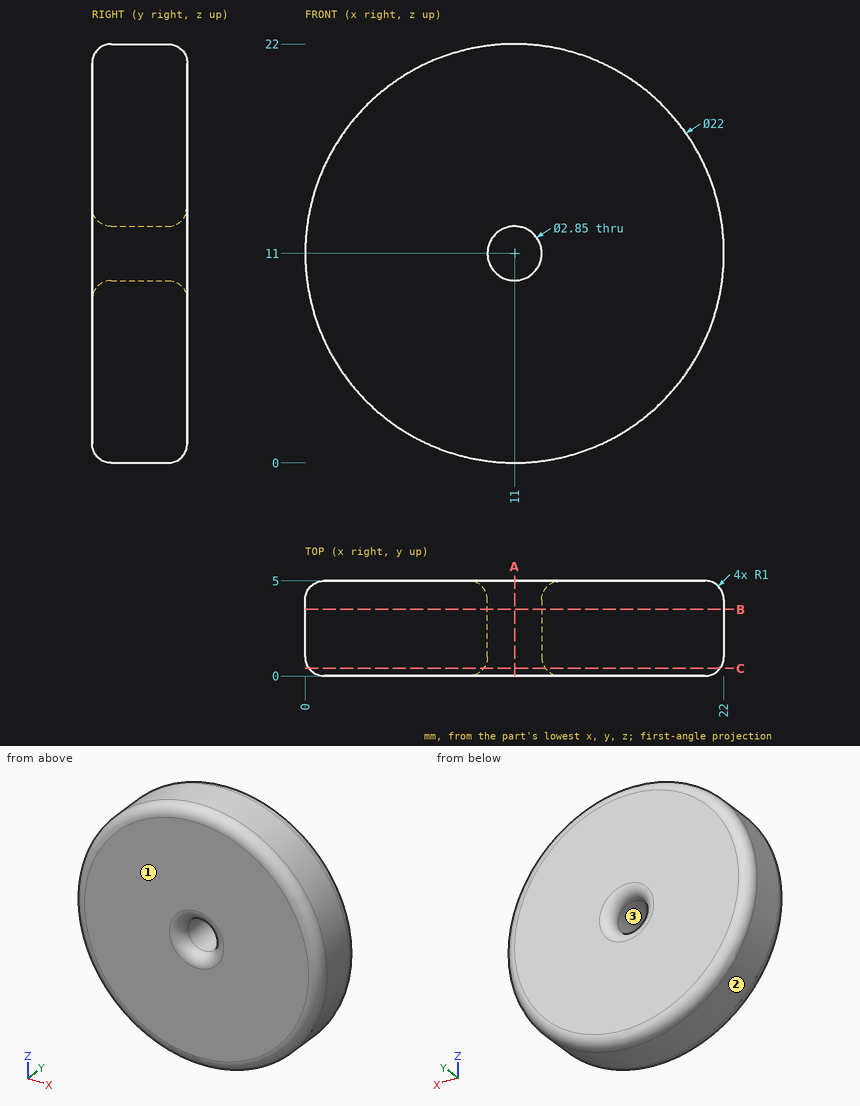
Here's the drawing with two shaded views (mm, measured from the low corner). I have some questions. Coordinates: 2 decimals unless noted, no trailing zeros. Loops run counter-clockwise (first coordinate to the right, second up) from the corner with the lowest first, then second, coordinate; pieces in that order, holes last.
Item 1: Suppose I cut it at A-A (x = 11). Please give me the cut outline in (y, z) (3 decimals).
Answers below:
outline: (0, 1) arc R1 ccw to (1, 0) - (4, 0) arc R1 ccw to (5, 1) - (5, 8.575) arc R1 ccw to (4, 9.575) - (1, 9.575) arc R1 ccw to (0, 8.575) - close; (0, 13.425) arc R1 ccw to (1, 12.425) - (4, 12.425) arc R1 ccw to (5, 13.425) - (5, 21) arc R1 ccw to (4, 22) - (1, 22) arc R1 ccw to (0, 21) - close
Item 2: Please list where these lines run through material, in increasing order: L1, parallel to X at y = 2.45, z = 10.5; L2, parallel to Z at x = 16.25, y = 3.5; L3, parallel to Z at x = 12, y = 2.
Answers below:
L1: x = 0.01 to 9.67, 12.33 to 21.99
L2: z = 1.33 to 20.67
L3: z = 0.05 to 9.98, 12.02 to 21.95
Item 3: Suppose I cut it at B-B (y = 3.5). Please give me the cut outline in (x, z) (3 decimals), then the cut area to 3 significant figures.
Answers below:
outline: circle Ø22 at (11, 11); hole circle Ø2.85 at (11, 11)
area: 374 mm2
Item 4: If we mould it in two halves opening along Z, with no side actions, what happens to the marked faces 1, 2 and 3? For each: released by +Z, released by -Z, zero draft, split by the parting line, or undercut.
Answers below:
face 1: zero draft
face 2: split by the parting line
face 3: undercut
Item 5: Suppose I cut it at C-C (y = 0.4). Please give me the cut outline in (x, z) (3 decimals).
Answers below:
outline: circle Ø21.6 at (11, 11); hole circle Ø3.25 at (11, 11)
Item 6: I'm going to push flat-ended pins straight in: pin 1 (1 mm diameter, centred on y = 1, z = 13.5, fed in from -X); pin 2 (1.5 mm diameter, centred on x = 17, y = 4, fed in from -Z); pin 3 (2 mm diameter, centred on x = 5.5, y = 1, fed in from -Z). Where does each tip first touch, or does it pass through?
Answers below:
pin 1: stops at x = 0.18
pin 2: stops at z = 1.33
pin 3: stops at z = 0.96
